The model under review builds one solid part; all positions refer to its coordinate system, in mm. Round coordinates to 2 decimals unless told otherwise and drop trailing zeros. Write each loop counter-clockwise with the first axis right and the second up, starting at its lowest first coordinate (ties: lowest second). Pieces come first, ordered by that corner, then holes. Notation, with made-up numbers: M 70,47.25 L 115,47.25 A4 ccw 115,54.25 Z; hole C 10.5,-35 d7. An arc over 180 degrees is marked long. Write item = value, one per line. Start each with the question number.
Item 1: For pin 1 Ø1 at (x, y) = (6.5, -1.5) entering from -Z; pin 2 Ø1.5 at (x, y) = (-6.5, -3) entering from -Z; pin 3 Ø12 at (x, y) = (-1, 7) entering from +Z; pin 4 Ø8.5 at (x, y) = (0, 0) entering from +Z, all flat-tipped, find the tip position at first contact; note any pin that passes through.
Item 2: Take a section at B-B, the plane x = 0. Give the boundary of the cut face in (y, z), plus the area to 3 significant figures.
Item 3: Take a section at A-A, the plane y = -2.5. Give the boundary of the cut face in (x, z), plus the area to 3 significant figures.
Item 4: Take a section at C-C, the plane z = 38.5. Give the boundary of the cut face in (x, y).
Item 5: To check wall thickness, follow line 1 along X through (y, z) = (0, 23.5); line 2 along Y through (x, z) = (4.5, 50). State the ranges of each line that lie inside material, in increasing order.
Item 6: Take a section at D-D, the plane z = 0.5. Give the boundary of the cut face in (x, y).
Autodesk Inventor part; units mm, degrees
ref_plane "Start Plane" through (0, 0, -8.6396) normal (0, 0, 1) x (1, 0, 0)
ref_plane "End Plane" through (0, 0, 70.8143) normal (0, 0, 1) x (1, 0, 0)
ref_plane "Work Plane4" through (6.5224, -8.4419, -6.1592) normal (-0.3057, 0.3957, -0.866) x (0.3025, 0.9028, 0.3057)
ref_plane "Start Plane" through (0, 0, -8.6396) normal (0, 0, 1) x (1, 0, 0)
ref_plane "End Plane" through (0, 0, 70.8143) normal (0, 0, 1) x (1, 0, 0)
sketch "Sketch" plane through (0, 0, 0) normal (0, 0, 1) x (1, 0, 0)
  circle A0 centre (0, 0) radius 6.9342
  circle A1 centre (0, 0) radius 10.668
  dimension "d0" = 21.336
  dimension "d1" = 3.7338
extrude "Body" add sketch "Sketch" along normal up to surface (79.4539 mm away) from surface at -8.6396
sketch "Sketch3" plane through (0, 0, 0) normal (0, 0, 1) x (1, 0, 0)
  line L0 (0, 0) -> (10, 0)
ref_plane "Work Plane3" through (0, 0, 0) normal (0, -1, 0) x (1, 0, 0)
sketch "Sketch4" plane through (0, 0, 0) normal (0, -1, 0) x (1, 0, 0)
  line L0 (-2, -8.6396) -> (12, -8.6396)
  line L1 (-2, 70.8143) -> (12, 70.8143)
  dimension "d7" = 79.4539
ref_plane "Work Plane4" through (6.5224, -8.4419, -6.1592) normal (-0.3057, 0.3957, -0.866) x (0.3025, 0.9028, 0.3057)
split "Split1" plane through (6.5224, -8.4419, -6.1592) removes the side toward (-0.3057, 0.3957, -0.866)
ref_plane "Work Plane5" through (6.5224, -8.4419, 70.9087) normal (-0.0922, 0.1193, 0.9886) x (0.9957, 0.0055, 0.0922)
split "Split2" plane through (6.5224, -8.4419, 70.9087) removes the side toward (-0.0922, 0.1193, 0.9886)
ref_plane "Work Plane6" through (-9.8011, -4.2125, 86.2321) normal (0.7776, 0.3342, 0.5327) x (0.6055, -0.1695, -0.7776)
split "Split3" plane through (-9.8011, -4.2125, 86.2321) removes the side toward (0.7776, 0.3342, 0.5327)
equation "\"d0\" = G_H"
equation "\"d1\" = G_T"
equation "\"d2\" = G_L"
equation "\"G_H\" = 21.336"
equation "\"G_T\" = 3.7338"
equation "\"G_L\" = 76.97342"
equation "\"G_OFFSET_START\" = 8.6396"
equation "\"G_OFFSET_END\" = 1.53222"
equation "\"d4\" = -G_OFFSET_START"
equation "\"d5\" = G_OFFSET_END + B_L"
equation "\"B_L\" = 69.28203"
properties part number "ANSI - 1/2 x 0.147 - 3.03" material "Steel, Mild"
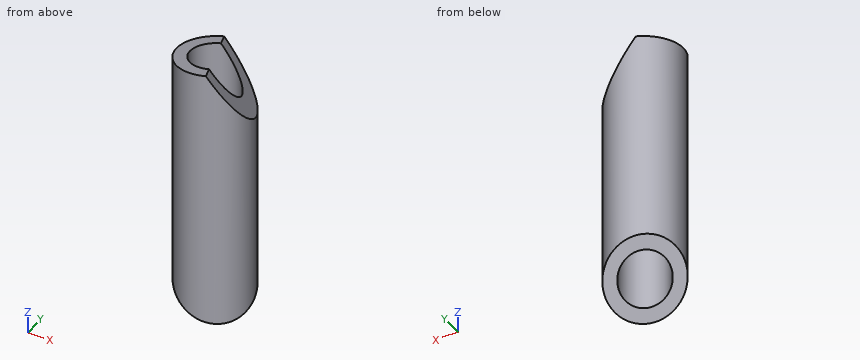
Response values:
q1.pin_1 = -3.27
q1.pin_2 = 0.49
q1.pin_3 = 68.3
q1.pin_4 = through
q2.outline = M -10.67,-4.87 L -6.93,-3.17 L -6.93,70.12 L -10.67,70.57 Z; M 6.93,3.17 L 10.67,4.88 L 10.67,62.59 L 6.93,64.93 Z
q2.area = 501 mm2
q3.outline = M -10.37,2.52 L -6.47,1.14 L -6.47,68.98 L -10.37,68.62 Z; M 6.47,-3.42 L 10.37,-4.8 L 10.37,55.71 L 6.47,61.41 Z
q3.area = 506 mm2
q4.outline = C 0,0 d21.34; hole C 0,0 d13.87
q5.line_1 = -10.67 to -6.93, 6.93 to 10.67
q5.line_2 = -9.67 to -5.28, 5.28 to 9.67
q6.outline = M -8.94,-5.82 A10.67 ccw long 7.89,7.19 L 4.92,4.89 A6.93 cw long -5.97,-3.52 Z
